Here's how the part is built. I have some questions about the finished solid (model axes, mm). A direction names the side the tool comes from. Round coordinates to 2 decimals unless told otherwise and drop trailing zeros. Loops run counter-clockwise (first coordinate to the right, second up) from the corner with the lowest first, then second, coordinate; pieces in that order, holes last. Notation, with made-up numbers: (43, -25) -> (75, -25) arc R13 ccw to (75, -8) -> close; hole circle Ø10 at (-29, 58). An arc over 180 degrees is marked (long way). One line per item, written item: value. Start each with the question number.
```python
from build123d import *

# Parameters (mm, degrees)
ESQUISSE1_R             = 3.5
ESQUISSE1_R_2           = 2.95
BOSS_EXTRU_1_DEPTH      = 4
ESQUISSE2_R             = 7.5
BOSS_EXTRU_2_DEPTH      = 1.5
ESQUISSE3_R             = 0.5
ENL_V_MAT_EXTRU_3_DEPTH = 2


with BuildPart() as part:
    # Esquisse1 → Boss.-Extru.1 (new body)
    with BuildSketch(Plane.XY):
        Circle(ESQUISSE1_R)
        Circle(ESQUISSE1_R_2, mode=Mode.SUBTRACT)
    extrude(amount=BOSS_EXTRU_1_DEPTH)

    # Esquisse2 → Boss.-Extru.2 (add)
    with BuildSketch(Plane(origin=(0, 0, 0), x_dir=(-1, 0, 0), z_dir=(0, 0, -1))):
        Circle(ESQUISSE2_R)
    extrude(amount=BOSS_EXTRU_2_DEPTH)

    # Esquisse3 → Enlèv. mat.-Extru.3 (cut)
    with BuildSketch(Plane(origin=(0, 0, -1.5), x_dir=(-1, 0, 0), z_dir=(0, 0, -1))):
        with Locations((0, 5)):
            Circle(ESQUISSE3_R)
        with Locations((5, 0)):
            Circle(ESQUISSE3_R)
        with Locations((0, -5)):
            Circle(ESQUISSE3_R)
        with Locations((-5, 0)):
            Circle(ESQUISSE3_R)
    extrude(amount=-ENL_V_MAT_EXTRU_3_DEPTH, mode=Mode.SUBTRACT)


solid = part.part
```
Q1. Will these pins go through, and if not, where does the flat tip stop? P1, Ø1.5, axis at x = -4.5, z = -0.5, coming from the +Y side; P2, Ø1, axis at x = 5.5, z = -0.5, coming from the -Y side.
Q2. I want a section at A-A on x = 0. Please give me the cut outline in (y, z), plus the area to 3 significant figures.
Q3. I want a section at B-B on z = 3.5. Please give me the cut outline in (x, y).
Q4. I want a section at C-C on x = -5. Please give me the cut outline in (y, z).
Q5. Which directions (+Z, -Z, +X, -X, +Y, -Y) give clear straight access to the entire face, cutting with the end or side of a thin tool? Please do faces 1 (the cylindrical face through (0.065, 5.496, -0.76)), 2 (the cylindrical face through (3.233, -1.341, 1.972)).
Q6. If we mould it in two halves opening along X, with no side actions, what happens to faces 3 (the cylindrical face through (5.4, -0.3, -0.8)), 4 (the cylindrical face through (7.493, 0.33, -0.74)), 5 (the flat face through (0, 0, -1.5))? For each: released by +X, released by -X, zero draft, split by the parting line, or undercut.
Q7. If I drill on line 1 along Y through (x, z) = (0, -0.6); line 2 along Y through (x, z) = (0, 1.1); line 3 along Z through (x, y) = (-3.75, -5), over which ranges is the centre line in solid material (lowest first)?
Answers below:
1. P1: stops at y = 6.5
1. P2: stops at y = -5.59
2. outline: (-7.5, -1.5) -> (-5.5, -1.5) -> (-5.5, 0) -> (-7.5, 0) -> close; (-4.5, -1.5) -> (4.5, -1.5) -> (4.5, 0) -> (3.5, 0) -> (3.5, 4) -> (2.95, 4) -> (2.95, 0) -> (-2.95, 0) -> (-2.95, 4) -> (-3.5, 4) -> (-3.5, 0) -> (-4.5, 0) -> close; (5.5, -1.5) -> (7.5, -1.5) -> (7.5, 0) -> (5.5, 0) -> close
2. area: 23.9 mm^2
3. outline: circle Ø7 at (0, 0); hole circle Ø5.9 at (0, 0)
4. outline: (-5.59, -1.5) -> (-0.5, -1.5) -> (-0.5, 0) -> (-5.59, 0) -> close; (0.5, -1.5) -> (5.59, -1.5) -> (5.59, 0) -> (0.5, 0) -> close
5. face 1: +Z, -Z
5. face 2: +Z
6. face 3: undercut
6. face 4: split by the parting line
6. face 5: zero draft
7. line 1: y = -7.5 to -5.5, -4.5 to 4.5, 5.5 to 7.5
7. line 2: y = -3.5 to -2.95, 2.95 to 3.5
7. line 3: z = -1.5 to 0
